For this review, take the finished solid that the model builds, in its own axes (mm). A direction names the side the tool comes from. Round coordinates to 2 decimals unless told otherwise and drop trailing zeros. Loops run counter-clockwise (first coordinate to the right, second up) from the corner with the lowest first, then second, coordinate; pieces in that order, holes last. Notation, with made-up numbers: (73, 71) -> (107, 71) arc R23 ccw to (107, 101) -> close; hole circle Ø4 at (66.5, 4.5). An arc over 180 degrees is marked (long way). One line per question, with ' | ' between items. Start each with the question number.
1. For pin 1 Ø2 at (x, y) = (2, 9.5) entering from -Z; pin 2 Ø1.5 at (y, z) = (3, 1) entering from +X, all flat-tipped, find the tip position at first contact; note any pin that passes through.
2. Consider section A-A (y = 2). Write out the cut boundary in (x, z).
3. Draft analysis for pull direction Z (two halves, no side actions). For faces 1 (the face through (-6.221, 0.128, 0.015)), 2 (the face through (-3.1, 0.13, 5.4)), 3 (the face through (0, 3, -6)), 4 (the face through (1.06, 9.13, 2.86)), state which applies: pulls with the +Z half, pulls with the -Z half, needs draft (parallel to the pull), parting line crosses it, or undercut.
4. Consider section B-B (y = 10). Write out the cut boundary in (x, z), and give its area (3 significant figures).
5. For faces 5 (the face through (-5.37, 11.92, -1.19)), 6 (the face through (-5.22, 2.96, 2.96)), list the 3-axis set-ups (+Z, -Z, +X, -X, +Y, -Y) from which the entire face can be reached by the end or side of a thin tool; tool diameter is ignored.
6. Wall thickness on line 1 along X through (y, z) = (9.75, 0); line 2 along X through (y, z) = (17.25, 0.75); line 3 along Z through (x, y) = (-2, 16.25): over which ranges is each line inside the solid? List them lowest first.
```python
from build123d import *

# Parameters (mm, degrees)
EXTRUDE_1_DEPTH     = 6
SKETCH_2_R          = 5.5
EXTRUDE_2_DEPTH     = 12
SKETCH_3_R          = 3
CUT_EXTRUDE_1_DEPTH = 21.199009877
SKETCH_4_OUTSIDE_W  = 55.636
SKETCH_4_OUTSIDE_H  = 53.78
SKETCH_4_OUTSIDE_R  = 6
CUT_EXTRUDE_2_DEPTH = 10
CUT_EXTRUDE_2_DRAFT = -60


with BuildPart() as part:
    # 草图1 → 凸台-拉伸1 (new body)
    with BuildSketch(Plane(origin=(0, 0, 0), x_dir=(1, 0, 0), z_dir=(0, 1, 0))):
        Polygon((6.92820323, 0), (3.464101615, 6), (-3.464101615, 6), (-6.92820323, 0), (-3.464101615, -6), (3.464101615, -6), align=None)
    extrude(amount=EXTRUDE_1_DEPTH)

    # 草图2 → 凸台-拉伸2 (add)
    with BuildSketch(Plane(origin=(0, 6, 0), x_dir=(1, 0, 0), z_dir=(0, 1, 0))):
        with Locations(Location((0, 0, 0), (0, 0, 270))):
            Circle(SKETCH_2_R)
    extrude(amount=EXTRUDE_2_DEPTH)

    # 草图3 → 切除-拉伸1 (cut, through all)
    with BuildSketch(Plane(origin=(0, 18, 0), x_dir=(1, 0, 0), z_dir=(0, 1, 0))):
        with Locations(Location((0.154901244, 0, 0), (0, 0, 270))):
            Circle(SKETCH_3_R)
    extrude(amount=-CUT_EXTRUDE_1_DEPTH, mode=Mode.SUBTRACT)


with BuildPart() as cut_extrude_2_tool:
    # 草图4 outside → 切除-拉伸2 (with draft: the straight prism first)
    with BuildSketch(Plane.XZ):
        Rectangle(SKETCH_4_OUTSIDE_W, SKETCH_4_OUTSIDE_H)
        Circle(SKETCH_4_OUTSIDE_R, mode=Mode.SUBTRACT)
    extrude(amount=-CUT_EXTRUDE_2_DEPTH)
    # 切除-拉伸2: the draft: its side faces are tilted about the plane it starts from
    cut_extrude_2_sides = [cut_extrude_2_tool.faces().sort_by_distance(p)[0] for p in [
        (0, 5, -26.89),
        (27.818, 5, 0),
        (0, 5, 26.89),
        (-27.818, 5, 0),
        (-6, 5, 0),
    ]]
    draft(cut_extrude_2_sides, Plane.XZ, CUT_EXTRUDE_2_DRAFT)


with BuildPart() as part_1:
    add(part.part)

    # 切除-拉伸2: cut by cut_extrude_2_tool
    add(cut_extrude_2_tool.part, mode=Mode.SUBTRACT)


solid = part_1.part
```
Answer block:
1) pin 1: stops at z = -5.41 | pin 2: stops at x = 6.78
2) outline: (-6.93, 0) -> (-3.46, -6) -> (3.46, -6) -> (6.93, 0) -> (3.46, 6) -> (-3.46, 6) -> close; hole circle Ø6 at (0.15, 0)
3) face 1: parting line crosses it | face 2: pulls with the +Z half | face 3: pulls with the -Z half | face 4: undercut
4) outline: circle Ø11 at (0, 0); hole circle Ø6 at (0.15, 0) | area: 66.8 mm2
5) face 5: +Y | face 6: +Z, -X, +Y, -Y
6) line 1: x = -5.5 to -2.85, 3.15 to 5.5 | line 2: x = -5.45 to -2.75, 3.06 to 5.45 | line 3: z = -5.12 to -2.09, 2.09 to 5.12
